```python
from build123d import *

# Parameters (mm, degrees)
BASE_DEPTH          = 2.5
BASE_PATTERN_COUNT  = 5
BASE_PATTERN_PITCH  = 2.54
CUT_DEPTH           = 12.768933682
CUT_DEPTH_BACK      = 12.768933682
SKETCH2_W           = 1.54
SKETCH2_H           = 0.44
SKETCH3_W           = 0.65
SKETCH3_H           = 0.65
PIN_CHAMFER_SIZE    = 0.15
PIN_CHAMFER_SIZE2   = 0.321676038
CHAMFER1_SIZE       = 0.15
CHAMFER1_SIZE2      = 0.321676038
PIN_START           = 2.215
PIN_PATTERN_DEPTH   = 0.65
PIN_START_2         = 4.755
PIN_PATTERN_2_DEPTH = 0.65
PIN_START_3         = 7.295
PIN_PATTERN_3_DEPTH = 0.65
PIN_START_4         = 9.835
PIN_PATTERN_4_DEPTH = 0.65
PIN_START_5         = -6.678323962
PIN_PATTERN_5_DEPTH = 7.678323962
PIN_START_6         = 2.5
PIN_PATTERN_6_DEPTH = 2.5


with BuildPart() as part:
    # Sketch1 → Base (new body)
    with BuildSketch(Plane(origin=(0, 0, 0), x_dir=(1, 0, 0), z_dir=(0, 1, 0))):
        Polygon((-1.27, 0.97), (-0.97, 1.27), (0.97, 1.27), (1.27, 0.97), (1.27, -0.97), (0.97, -1.27), (-0.97, -1.27), (-1.27, -0.97), align=None)
    base = extrude(amount=BASE_DEPTH)

    # Base_Pattern: Base ×5
    with Locations(*[(i * BASE_PATTERN_PITCH, 0, 0) for i in range(1, BASE_PATTERN_COUNT)]):
        add(base)

    # Sketch2 → Cut (cut, two sides: drawn at the far end of the back side and taken through both)
    with BuildSketch(Plane(origin=(0, 0, 0), x_dir=(0, 0, -1), z_dir=(1, 0, 0)).offset(-CUT_DEPTH_BACK)):
        with Locations((0, 0.22)):
            Rectangle(SKETCH2_W, SKETCH2_H)
    extrude(amount=CUT_DEPTH + CUT_DEPTH_BACK, mode=Mode.SUBTRACT)

    # Sweep1: sweep along a path in Sketch4
    with BuildLine(Plane(origin=(0, 0, 0), x_dir=(0, 0, -1), z_dir=(1, 0, 0))) as sweep1_path:
        Line((0, -3), (0, 3.25))
        ThreePointArc((0, 3.25), (0.219669914, 3.780330086), (0.75, 4))
        Line((0.75, 4), (7, 4))
    # Sketch3 → Sweep1 (sweep)
    with BuildSketch(Plane(origin=(0, -3, 0), x_dir=(1, 0, 0), z_dir=(0, 1, 0))):
        Rectangle(SKETCH3_W, SKETCH3_H)
    sweep(path=sweep1_path.line)

    # Pin Chamfer
    pin_chamfer_edges = [part.edges().sort_by_distance(p)[0] for p in [
        (0.325, -3, 0),
        (0, -3, -0.325),
        (-0.325, -3, 0),
        (0, -3, 0.325),
    ]]
    pin_chamfer_side = [part.faces().sort_by_distance(p)[0] for p in [
        (0, -3, 0),
    ]]
    chamfer(pin_chamfer_edges, length=PIN_CHAMFER_SIZE, length2=PIN_CHAMFER_SIZE2, reference=pin_chamfer_side[0])

    # Chamfer1
    chamfer1_edges = [part.edges().sort_by_distance(p)[0] for p in [
        (-0.325, 4, -7),
        (0, 4.325, -7),
        (0.325, 4, -7),
        (0, 3.675, -7),
    ]]
    chamfer1_side = [part.faces().sort_by_distance(p)[0] for p in [
        (0, 4, -7),
    ]]
    chamfer(chamfer1_edges, length=CHAMFER1_SIZE, length2=CHAMFER1_SIZE2, reference=chamfer1_side[0])

    # Pin Pattern: read off the stored shape, not the designer's step
    # Pin Pattern outline → Pin Pattern (add)
    with BuildSketch(Plane.YZ.offset(PIN_START)):
        Polygon((-2.678323962, 0.325), (-3, 0.175), (-3, -0.175), (-2.678323962, -0.325), (0.44, -0.325), (0.44, 0.325), align=None)
        with BuildLine():
            Line((2.5, -0.325), (3.25, -0.325))
            ThreePointArc((3.25, -0.325), (3.550520382, -0.449479618), (3.675, -0.75))
            Line((3.675, -0.75), (3.675, -6.678323962))
            Line((3.675, -6.678323962), (3.825, -7))
            Line((3.825, -7), (4.175, -7))
            Line((4.175, -7), (4.325, -6.678323962))
            Line((4.325, -6.678323962), (4.325, -0.75))
            ThreePointArc((4.325, -0.75), (4.01013979, 0.01013979), (3.25, 0.325))
            Line((3.25, 0.325), (2.5, 0.325))
            Line((2.5, 0.325), (2.5, -0.325))
        make_face()
    extrude(amount=PIN_PATTERN_DEPTH)

    # Pin Pattern 2 outline → Pin Pattern 2 (add)
    with BuildSketch(Plane.YZ.offset(PIN_START_2)):
        Polygon((-2.678323962, 0.325), (-3, 0.175), (-3, -0.175), (-2.678323962, -0.325), (0.44, -0.325), (0.44, 0.325), align=None)
        with BuildLine():
            Line((2.5, -0.325), (3.25, -0.325))
            ThreePointArc((3.25, -0.325), (3.550520382, -0.449479618), (3.675, -0.75))
            Line((3.675, -0.75), (3.675, -6.678323962))
            Line((3.675, -6.678323962), (3.825, -7))
            Line((3.825, -7), (4.175, -7))
            Line((4.175, -7), (4.325, -6.678323962))
            Line((4.325, -6.678323962), (4.325, -0.75))
            ThreePointArc((4.325, -0.75), (4.01013979, 0.01013979), (3.25, 0.325))
            Line((3.25, 0.325), (2.5, 0.325))
            Line((2.5, 0.325), (2.5, -0.325))
        make_face()
    extrude(amount=PIN_PATTERN_2_DEPTH)

    # Pin Pattern 3 outline → Pin Pattern 3 (add)
    with BuildSketch(Plane.YZ.offset(PIN_START_3)):
        Polygon((-2.678323962, 0.325), (-3, 0.175), (-3, -0.175), (-2.678323962, -0.325), (0.44, -0.325), (0.44, 0.325), align=None)
        with BuildLine():
            Line((2.5, -0.325), (3.25, -0.325))
            ThreePointArc((3.25, -0.325), (3.550520382, -0.449479618), (3.675, -0.75))
            Line((3.675, -0.75), (3.675, -6.678323962))
            Line((3.675, -6.678323962), (3.825, -7))
            Line((3.825, -7), (4.175, -7))
            Line((4.175, -7), (4.325, -6.678323962))
            Line((4.325, -6.678323962), (4.325, -0.75))
            ThreePointArc((4.325, -0.75), (4.01013979, 0.01013979), (3.25, 0.325))
            Line((3.25, 0.325), (2.5, 0.325))
            Line((2.5, 0.325), (2.5, -0.325))
        make_face()
    extrude(amount=PIN_PATTERN_3_DEPTH)

    # Pin Pattern 4 outline → Pin Pattern 4 (add)
    with BuildSketch(Plane.YZ.offset(PIN_START_4)):
        Polygon((-2.678323962, 0.325), (-3, 0.175), (-3, -0.175), (-2.678323962, -0.325), (0.44, -0.325), (0.44, 0.325), align=None)
        with BuildLine():
            Line((2.5, -0.325), (3.25, -0.325))
            ThreePointArc((3.25, -0.325), (3.550520382, -0.449479618), (3.675, -0.75))
            Line((3.675, -0.75), (3.675, -6.678323962))
            Line((3.675, -6.678323962), (3.825, -7))
            Line((3.825, -7), (4.175, -7))
            Line((4.175, -7), (4.325, -6.678323962))
            Line((4.325, -6.678323962), (4.325, -0.75))
            ThreePointArc((4.325, -0.75), (4.01013979, 0.01013979), (3.25, 0.325))
            Line((3.25, 0.325), (2.5, 0.325))
            Line((2.5, 0.325), (2.5, -0.325))
        make_face()
    extrude(amount=PIN_PATTERN_4_DEPTH)

    # Pin Pattern 5 outline → Pin Pattern 5 (cut)
    with BuildSketch(Plane.XY.offset(PIN_START_5)):
        Polygon((2.865, -2.678323962), (2.715, -3), (2.865, -3), align=None)
        Polygon((2.365, -3), (2.215, -2.678323962), (2.215, -3), align=None)
        Polygon((5.405, -2.678323962), (5.255, -3), (5.405, -3), align=None)
        Polygon((4.905, -3), (4.755, -2.678323962), (4.755, -3), align=None)
        Polygon((7.945, -2.678323962), (7.795, -3), (7.945, -3), align=None)
        Polygon((7.445, -3), (7.295, -2.678323962), (7.295, -3), align=None)
        Polygon((10.485, -2.678323962), (10.335, -3), (10.485, -3), align=None)
        Polygon((9.985, -3), (9.835, -2.678323962), (9.835, -3), align=None)
    extrude(amount=PIN_PATTERN_5_DEPTH, mode=Mode.SUBTRACT)

    # Pin Pattern 6 outline → Pin Pattern 6 (cut)
    with BuildSketch(Plane(origin=(0, 0, 0), x_dir=(1, 0, 0), z_dir=(0, 1, 0)).offset(PIN_START_6)):
        Polygon((2.865, 7), (2.715, 7), (2.865, 6.678323962), align=None)
        Polygon((2.215, 6.678323962), (2.365, 7), (2.215, 7), align=None)
        Polygon((5.405, 7), (5.255, 7), (5.405, 6.678323962), align=None)
        Polygon((4.755, 6.678323962), (4.905, 7), (4.755, 7), align=None)
        Polygon((7.945, 7), (7.795, 7), (7.945, 6.678323962), align=None)
        Polygon((7.295, 6.678323962), (7.445, 7), (7.295, 7), align=None)
        Polygon((10.485, 7), (10.335, 7), (10.485, 6.678323962), align=None)
        Polygon((9.835, 6.678323962), (9.985, 7), (9.835, 7), align=None)
    extrude(amount=PIN_PATTERN_6_DEPTH, mode=Mode.SUBTRACT)


solid = part.part
```
Work out the finished part from the listing and answer in its coordinate system (mm). A direction names the side the tool comes from. Coordinates: 2 decimals unless noted, no trailing zeros. Write each loop counter-clockwise with the first axis right and the second up, starting at its lowest first coordinate (ties: lowest second). Pieces come first, ordered by that corner, then holes. Notation, with made-up numbers: (64, -33) - (94, -33) arc R8 cw to (94, -22) - close; hole circle Ø10 at (-10, 56). An arc over 180 degrees is marked (long way). Answer as a JSON object with one key per item and string values.
Q1. Given pin 1 Ø0.6 at (x, z) = (4, 1) entering from -Y; pin 2 Ø0.6 at (x, y) = (8, 1) entering from -Z; pin 3 Ø0.5 at (y, z) = (-0.5, 0) entering from -X (3 decimals); pin 4 Ø2 at (y, z) = (-2, -3) entering from -X, each flat-ended and moving along its own axis, determine where each tip first touches the part or whether it passes through.
Results list:
{"pin 1": "stops at y = 0", "pin 2": "stops at z = -1.27", "pin 3": "stops at x = -0.325", "pin 4": "passes through"}
Q2. Which of the six approach directions +Z, -Z, +X, -X, +Y, -Y give full straight-line access (tool end or side, diameter ignored) to faces 1 (the flat face through (10, 1, 1.27)), 2 (the flat face through (0, 1, -1.27)), 3 (the flat face through (7.295, 4, -2))?
Results list:
{"face 1": "+Z, +X, -X, +Y, -Y", "face 2": "-Z, +X, -X, -Y", "face 3": "+Z, -Z, +Y"}
Q3. Consider L1, parallel to X at y = 4.25, z = -3 (3 decimals); L2, parallel to Z at x = 2, y = 0.25; L3, parallel to Y at x = 0, z = -6.5 (3 decimals). Determine where each line is inside the solid, lowest interval first. Write a range as from..to.
Results list:
{"L1": "x = -0.325..0.325, 2.215..2.865, 4.755..5.405, 7.295..7.945, 9.835..10.485", "L2": "z = -1.27..-0.77, 0.77..1.27", "L3": "y = 3.675..4.325"}
Q4. For a pull along X with two mould halves and no side action, classify faces 4 (the cylindrical face through (2.54, 4.02, 0)), 5 (the flat face through (11.43, 2, 0)), 6 (the flat face through (-0.325, 4, -2)), 7 (the flat face through (2.215, 4, -2)) as pulls with the +X half, pulls with the -X half, needs draft (parallel to the pull), parting line crosses it, or undercut.
Results list:
{"face 4": "needs draft", "face 5": "pulls with the +X half", "face 6": "pulls with the -X half", "face 7": "undercut"}
Q5. Find section A-A (y = -1.5). Write down the section's boundary in (x, z) (3 decimals).
Results list:
{"outline": "(-0.325, -0.325) - (0.325, -0.325) - (0.325, 0.325) - (-0.325, 0.325) - close; (2.215, -0.325) - (2.865, -0.325) - (2.865, 0.325) - (2.215, 0.325) - close; (4.755, -0.325) - (5.405, -0.325) - (5.405, 0.325) - (4.755, 0.325) - close; (7.295, -0.325) - (7.945, -0.325) - (7.945, 0.325) - (7.295, 0.325) - close; (9.835, -0.325) - (10.485, -0.325) - (10.485, 0.325) - (9.835, 0.325) - close"}
Q6. Find section C-C (z = -2.25). Write down the section's boundary in (x, y) (3 decimals).
Results list:
{"outline": "(-0.325, 3.675) - (0.325, 3.675) - (0.325, 4.325) - (-0.325, 4.325) - close; (2.215, 3.675) - (2.865, 3.675) - (2.865, 4.325) - (2.215, 4.325) - close; (4.755, 3.675) - (5.405, 3.675) - (5.405, 4.325) - (4.755, 4.325) - close; (7.295, 3.675) - (7.945, 3.675) - (7.945, 4.325) - (7.295, 4.325) - close; (9.835, 3.675) - (10.485, 3.675) - (10.485, 4.325) - (9.835, 4.325) - close"}
Q7. Find section B-B (x = 10.75). Write down the section's boundary in (y, z).
Results list:
{"outline": "(0, -1.27) - (2.5, -1.27) - (2.5, 1.27) - (0, 1.27) - (0, 0.77) - (0.44, 0.77) - (0.44, -0.77) - (0, -0.77) - close"}
